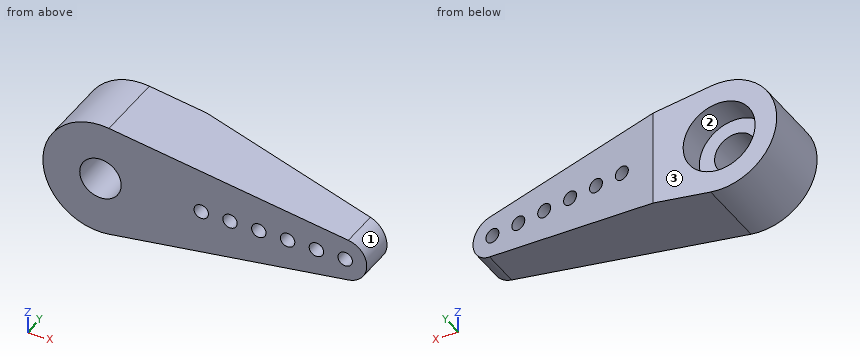
```python
from build123d import *

# Parameters (mm, degrees)
EXTRUDE_1_DEPTH          = 10
CUT_EXTRUDE_1_DEPTH      = 40.153543901
CUT_EXTRUDE_1_DEPTH_BACK = 40.153543901
SKETCH_4_R               = 5
CUT_EXTRUDE_2_DEPTH      = 4
SKETCH_5_R               = 2.88
CUT_EXTRUDE_3_DEPTH      = 6
SKETCH_6_R               = 1
CUT_EXTRUDE_4_DEPTH      = 40.153543901


with BuildPart() as part:
    # Эскиз1 → Бобышка-Вытянуть1 (new body)
    with BuildSketch(Plane(origin=(0, 0, 0), x_dir=(1, 0, 0), z_dir=(0, 1, 0))):
        with BuildLine():
            Line((1.176470588, 7.913021986), (34.441176471, 2.967383245))
            ThreePointArc((34.441176471, 2.967383245), (37, 0), (34.441176471, -2.967383245))
            Line((34.441176471, -2.967383245), (1.176470588, -7.913021986))
            ThreePointArc((1.176470588, -7.913021986), (-8, 0), (1.176470588, 7.913021986))
        make_face()
    extrude(amount=EXTRUDE_1_DEPTH)

    # Эскиз3 → Вырез-Вытянуть1 (cut, two sides: drawn at the far end of the back side and taken through both)
    with BuildSketch(Plane.XY.offset(-CUT_EXTRUDE_1_DEPTH_BACK)):
        Polygon((37, 5), (9.176470588, 10), (37, 10), align=None)
    extrude(amount=CUT_EXTRUDE_1_DEPTH + CUT_EXTRUDE_1_DEPTH_BACK, mode=Mode.SUBTRACT)

    # Эскиз4 → Вырез-Вытянуть2 (cut)
    with BuildSketch(Plane(origin=(0, 10, 0), x_dir=(1, 0, 0), z_dir=(0, 1, 0))):
        with Locations(Location((0, 0, 0), (0, 0, 270))):
            Circle(SKETCH_4_R)
    extrude(amount=-CUT_EXTRUDE_2_DEPTH, mode=Mode.SUBTRACT)

    # Эскиз5 → Вырез-Вытянуть3 (cut)
    with BuildSketch(Plane(origin=(0, 6, 0), x_dir=(1, 0, 0), z_dir=(0, 1, 0))):
        with Locations(Location((0, 0, 0), (0, 0, 270))):
            Circle(SKETCH_5_R)
    extrude(amount=-CUT_EXTRUDE_3_DEPTH, mode=Mode.SUBTRACT)

    # Эскиз6 → Вырез-Вытянуть4 (cut, through all)
    with BuildSketch(Plane.XZ):
        with Locations(Location((34, 0, 0), (0, 0, 270))):
            Circle(SKETCH_6_R)
        with Locations(Location((30, 0, 0), (0, 0, 270))):
            Circle(SKETCH_6_R)
        with Locations(Location((26, 0, 0), (0, 0, 270))):
            Circle(SKETCH_6_R)
        with Locations(Location((22, 0, 0), (0, 0, 270))):
            Circle(SKETCH_6_R)
        with Locations(Location((18, 0, 0), (0, 0, 270))):
            Circle(SKETCH_6_R)
        with Locations(Location((14, 0, 0), (0, 0, 270))):
            Circle(SKETCH_6_R)
    extrude(amount=-CUT_EXTRUDE_4_DEPTH, mode=Mode.SUBTRACT)


solid = part.part
```
Here's how the part is built. I have some questions about the finished solid (model axes, mm). Face numbers are marked on the shaded views. Round coordinates to 2 decimals unless told otherwise and drop trailing zeros. Write each loop counter-clockwise with the first axis right and the second up, starting at its lowest first coordinate (ties: lowest second). Pieces come first, ordered by that corner, then holes.
Q1. If we section it at A-A on x = 18: Write out the boundary of the cut face in (y, z).
Q2. If we section it at B-B on z = 2: Write out the boundary of the cut face in (x, y).
Q3. Please list where these lines run through material, in increasing order: probe 1 along Z at (x, y) = (14, 4.75); probe 2 along Y at (x, z) = (-3, -2.25); probe 3 along Z at (x, y) = (29.5, 3.5).
Q4. If we section it at D-D on x = 34: Write out the boundary of the cut face in (y, z).
Q5. If we mould it in two halves opening along X, with no side actions, what happens to the marked faces 1, 2 and 3? For each: +X half, -X half, draft (parallel to the pull), parting line (faces both ways), or undercut.
Q6. If we section it at C-C on z = -4.5: Write out the boundary of the cut face in (x, y).
Q7. Will these pins go through, and if not, where does the flat tip stop? P1, Ø8, axis at x = 19, z = 1, coming from the +Y side; P2, Ø1, axis at y = 1.5, z = -4, coming from the -X side; P3, Ø4, axis at x = 28.5, z = -2, coming from the +Y side.
Answer below:
1. outline: (0, -5.41) - (8.41, -5.41) - (8.41, -1) - (0, -1) - close; (0, 1) - (8.41, 1) - (8.41, 5.41) - (0, 5.41) - close
2. outline: (-7.75, 0) - (-2.07, 0) - (-2.07, 6) - (-4.58, 6) - (-4.58, 10) - (-7.75, 10) - close; (2.07, 0) - (36.24, 0) - (36.24, 5.14) - (9.18, 10) - (4.58, 10) - (4.58, 6) - (2.07, 6) - close
3. probe 1: z = -6.01 to -1, 1 to 6.01
3. probe 2: y = 0 to 6
3. probe 3: z = -3.7 to -0.87, 0.87 to 3.7
4. outline: (0, -3.03) - (5.54, -3.03) - (5.54, -1) - (0, -1) - close; (0, 1) - (5.54, 1) - (5.54, 3.03) - (0, 3.03) - close
5. face 1: +X half
5. face 2: undercut
5. face 3: draft
6. outline: (-6.61, 0) - (24.13, 0) - (24.13, 7.31) - (9.18, 10) - (2.18, 10) - (2.18, 6) - (-2.18, 6) - (-2.18, 10) - (-6.61, 10) - close
7. P1: stops at y = 8.95
7. P2: stops at x = -7.19
7. P3: stops at y = 6.89
